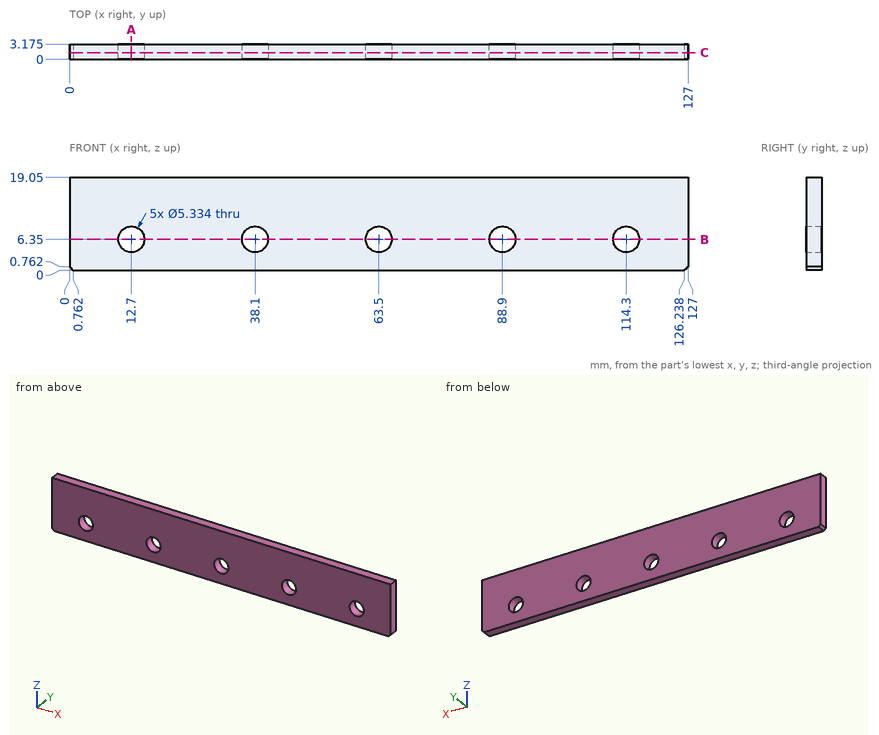
Part print with two shaded views. Sizes in mm from the minimum x, y, z corner. Round coordinates to 2 decimals unless told otherwise and drop trailing zeros. Order: outer loops, then holes, each group sorted by start corner. A loop starts at its lowest first (then second) coordinate and runs counter-clockwise, first axis right, second up. Notation, with made-up numbers: M -32,47.25 L 4,47.25 A15 ccw 4,59.25 Z; hole C -8.5,42.25 d3. An arc over 180 degrees is marked long. Use CSV: the item, a comma, the result in double quotes. Start each with the question number.
(1) Cut at C-C on y = 1.4. List the corners of the cut face in (x, z), then the cut area to 3 significant figures.
(2) Flat gauge pins, fed straight in: P1, Ø8.5, axis at x = 114.3, z = 6.35, coming from the -Y side; P2, Ø4.5, axis at x = 38.1, z = 6.35, coming from the +Y side. Where does each tip first touch, or does it go through?
(3) Cut at B-B on z = 6.35. List the corners of the cut face in (x, y) (3 decimals).
(4) Drill centre lines: probe 1 along Z at (x, y) = (114.3, 0.7); probe 2 along X at (y, z) = (1, 7.25); probe 3 along X at (y, z) = (1.4, 4.5). Where is each one in solid material? Low to high.
(5) Cut at A-A on x = 12.7. List the corners of the cut face in (y, z) (3 decimals).
Findings:
1,outline,"M 0,0.76 L 0.76,0 L 126.24,0 L 127,0.76 L 127,19.05 L 0,19.05 Z; hole C 12.7,6.35 d5.33; hole C 38.1,6.35 d5.33; hole C 63.5,6.35 d5.33; hole C 88.9,6.35 d5.33; hole C 114.3,6.35 d5.33"
1,area,"2,310 mm^2"
2,P1,"stops at y = 0"
2,P2,"passes through"
3,outline,"M 0,0 L 10.033,0 L 10.033,3.175 L 0,3.175 Z; M 15.367,0 L 35.433,0 L 35.433,3.175 L 15.367,3.175 Z; M 40.767,0 L 60.833,0 L 60.833,3.175 L 40.767,3.175 Z; M 66.167,0 L 86.233,0 L 86.233,3.175 L 66.167,3.175 Z; M 91.567,0 L 111.633,0 L 111.633,3.175 L 91.567,3.175 Z; M 116.967,0 L 127,0 L 127,3.175 L 116.967,3.175 Z"
4,probe 1,"z = 0 to 3.68, 9.02 to 19.05"
4,probe 2,"x = 0 to 10.19, 15.21 to 35.59, 40.61 to 60.99, 66.01 to 86.39, 91.41 to 111.79, 116.81 to 127"
4,probe 3,"x = 0 to 10.78, 14.62 to 36.18, 40.02 to 61.58, 65.42 to 86.98, 90.82 to 112.38, 116.22 to 127"
5,outline,"M 0,0 L 3.175,0 L 3.175,3.683 L 0,3.683 Z; M 0,9.017 L 3.175,9.017 L 3.175,19.05 L 0,19.05 Z"
